from build123d import *

# Parameters (mm, degrees)
SKETCH1_R                                         = 60.625
SKETCH1_R_2                                       = 45
BOSS_EXTRUDE1_DEPTH                               = 4
SKETCH2_R                                         = 49
SKETCH2_R_2                                       = 45
BOSS_EXTRUDE2_DEPTH                               = 52
SKETCH3_W                                         = 8
SKETCH3_H                                         = 38
BOSS_EXTRUDE3_DEPTH                               = 13
SKETCH5_W                                         = 10
SKETCH5_H                                         = 24
CUT_EXTRUDE1_DEPTH                                = 23
SKETCH6_R                                         = 5
CUT_EXTRUDE2_DEPTH                                = 60
SKETCH7_R                                         = 1.3
CUT_EXTRUDE3_DEPTH                                = 7.2
BOSS_EXTRUDE4_DEPTH                               = 4
CSK_FOR_0_FLAT_HEAD_MACHINE_SCREW_100_D           = 1.778
CSK_FOR_0_FLAT_HEAD_MACHINE_SCREW_100_CSINK_D     = 3.0226
CSK_FOR_0_FLAT_HEAD_MACHINE_SCREW_100_CSINK_ANGLE = 100
FILLET1_R                                         = 1


with BuildPart() as part:
    # Sketch1 → Boss-Extrude1 (new body)
    with BuildSketch(Plane(origin=(0, 0, 0), x_dir=(1, 0, 0), z_dir=(0, 1, 0))):
        with Locations(Location((0, 0, 0), (0, 0, 270))):
            Circle(SKETCH1_R)
        with Locations(Location((0, 0, 0), (0, 0, 270))):
            Circle(SKETCH1_R_2, mode=Mode.SUBTRACT)
    extrude(amount=BOSS_EXTRUDE1_DEPTH)

    # Sketch2 → Boss-Extrude2 (add)
    with BuildSketch(Plane(origin=(0, 4, 0), x_dir=(1, 0, 0), z_dir=(0, 1, 0))):
        with Locations(Location((0, 0, 0), (0, 0, 90))):
            Circle(SKETCH2_R)
        with Locations(Location((0, 0, 0), (0, 0, 270))):
            Circle(SKETCH2_R_2, mode=Mode.SUBTRACT)
    extrude(amount=BOSS_EXTRUDE2_DEPTH)

    # Sketch3 → Boss-Extrude3 (add, symmetric)
    with BuildSketch(Plane(origin=(0, 0, 0), x_dir=(0, 0, -1), z_dir=(1, 0, 0))):
        Polygon((-45, 38), (-31.75, 38), (-31.75, 30), (-45, 16.75), align=None)
        with Locations((15.25, 19)):
            Rectangle(SKETCH3_W, SKETCH3_H)
    extrude(amount=BOSS_EXTRUDE3_DEPTH, both=True)


with BuildPart() as boss_extrude3_piece_1:
    # of the separate pieces the step leaves, piece 1, a body of its own (boss_extrude3_pieces)
    add(part.part.solids().sort_by_distance((0, 0, 60.625))[0])

    # Sketch6 → Cut-Extrude2 (cut)
    with BuildSketch(Plane.XY.offset(-11.25)):
        with Locations(Location((0, 14, 0), (0, 0, 90))):
            Circle(SKETCH6_R)
    extrude(amount=-CUT_EXTRUDE2_DEPTH, mode=Mode.SUBTRACT)


with BuildPart() as boss_extrude3_piece_2:
    # of the separate pieces the step leaves, piece 2, a body of its own (boss_extrude3_pieces)
    add(part.part.solids().sort_by_distance((-13, 0, -19.25))[0])

    # Sketch5 → Cut-Extrude1 (cut)
    with BuildSketch(Plane.XY.offset(-11.25)):
        with Locations((0, 17)):
            Rectangle(SKETCH5_W, SKETCH5_H)
    extrude(amount=-CUT_EXTRUDE1_DEPTH, mode=Mode.SUBTRACT)


with BuildPart() as cut_extrude3_tool:
    # Sketch7 → Cut-Extrude3 (new body)
    with BuildSketch(Plane(origin=(0, 38, 0), x_dir=(1, 0, 0), z_dir=(0, 1, 0))):
        with Locations(Location((-5, 13.75, 0), (0, 0, 270))):
            Circle(SKETCH7_R)
        with Locations(Location((5, 13.75, 0), (0, 0, 270))):
            Circle(SKETCH7_R)
        with Locations(Location((5, -34.25, 0), (0, 0, 270))):
            Circle(SKETCH7_R)
        with Locations(Location((-5, -34.25, 0), (0, 0, 270))):
            Circle(SKETCH7_R)
    extrude(amount=-CUT_EXTRUDE3_DEPTH)


with BuildPart() as boss_extrude3_piece_1_1:
    add(boss_extrude3_piece_1.part)

    # Cut-Extrude3: cut by cut_extrude3_tool
    add(cut_extrude3_tool.part, mode=Mode.SUBTRACT)



with BuildPart() as boss_extrude3_piece_2_1:
    add(boss_extrude3_piece_2.part)

    # Cut-Extrude3: cut by cut_extrude3_tool
    add(cut_extrude3_tool.part, mode=Mode.SUBTRACT)


with BuildPart() as boss_extrude3_piece_1_2:
    add(boss_extrude3_piece_1_1.part)

    add(boss_extrude3_piece_2_1.part)  # Boss-Extrude4 merges Boss-Extrude3 piece 2
    # Sketch8 → Boss-Extrude4 (add)
    with BuildSketch(Plane.XZ):
        with BuildLine():
            Line((13, -11.25), (-13, -11.25))
            Line((-13, -11.25), (-37.248431585, -25.249838503))
            ThreePointArc((-37.248431585, -25.249838503), (0, -45), (37.248431585, -25.249838503))
            Line((37.248431585, -25.249838503), (13, -11.25))
        make_face()
        with BuildLine():
            Line((19.516660498, -24.25), (24.906460381, -27.361802413))
            ThreePointArc((24.906460381, -27.361802413), (0, -37), (-24.906460381, -27.361802413))
            Line((-24.906460381, -27.361802413), (-19.516660498, -24.25))
            Line((-19.516660498, -24.25), (19.516660498, -24.25))
        make_face(mode=Mode.SUBTRACT)
    extrude(amount=-BOSS_EXTRUDE4_DEPTH)

    # CSK for #0 Flat Head Machine Screw (100)1 (through all)
    with Locations(Plane(origin=(0, 4, 0), x_dir=(1, 0, 0), z_dir=(0, 1, 0))):
        with Locations((-35, 42), (35, 42), (35, -42), (-35, -42)):
            CounterSinkHole(CSK_FOR_0_FLAT_HEAD_MACHINE_SCREW_100_D / 2, CSK_FOR_0_FLAT_HEAD_MACHINE_SCREW_100_CSINK_D / 2, counter_sink_angle=CSK_FOR_0_FLAT_HEAD_MACHINE_SCREW_100_CSINK_ANGLE)

    # Fillet1
    fillet1_edges = [boss_extrude3_piece_1_2.edges().sort_by_distance(p)[0] for p in [
        (0, 4, 49),
    ]]
    fillet(fillet1_edges, radius=FILLET1_R)


solid = boss_extrude3_piece_1_2.part
Read the model definition and answer for the solid it produces. Units are mm, in the model's axes. A direction names the side the tool comes from. Round coordinates to 2 decimals unless told otherwise and drop trailing zeros. Loops run counter-clockwise (first coordinate to the right, second up) from the corner with the lowest first, then second, coordinate; pieces in that order, holes last.
Q1. Section A-A on y = 20.5 is taken. Write down the section's boundary in (x, z), and give its area (3 significant figures).
Q2. Which of the six approach directions +Z, -Z, +X, -X, +Y, -Y give full straight-line access (tool end or side, diameter ignored) to faces 1 (the face through (0, 9, -47)), 2 (the face through (5, 17, -15)), 3 (the face through (13, 21, -15)), 4 (the face through (-22.2, 2, -25.8))?
Q3. Each of these flat-tipped pins is pushed along its axis until it touches: pin 1 (14.5 mm diameter, centred on x = -6, z = 36.5, fed in from +Y); pin 2 (3.5 mm diameter, centred on y = 24.5, z = 35, fed in from +X); pin 3 (2 mm diameter, centred on y = 17.5, z = 18, fed in from -X). Where does it stop, or does it pass through?
Q4. Determine the mould class of faces 5 (the face through (-36.9, 2, -48.1)), 6 (the face through (22, 56, -40)), 7 (the face through (-13, 21, -15)) for opening direction X: released by +X, released by -X, zero draft, split by the parting line, or undercut.
Q5. Section D-D on y = 47 is taken. Write down the section's boundary in (x, z).
Q6. Section B-B on z = 0 is taken. Write down the section's boundary in (x, y) (3 decimals).
Q7. Section C-C on y = 12.5 is taken. Write down the section's boundary in (x, z).
Q8. Consider probe 1 along Z at (x, y) = (-10.5, 17.5); probe 2 along X at (y, z) = (2.3, -42); probe 3 along Y at (x, z) = (-1, -15.5). Determine where each line is inside the solid, lowest interval first.
Output:
1. outline: circle Ø98 at (0, 0); (-13, -19.25) - (-5, -19.25) - (-5, -11.25) - (-13, -11.25) - close; (5, -19.25) - (13, -19.25) - (13, -11.25) - (5, -11.25) - close; hole (-13, 41.25) - (-13, 43.08) arc R45 ccw (long way) to (13, 43.08) - (13, 41.25) - close
1. area: 1,390 mm2
2. face 1: -Z
2. face 2: none
2. face 3: +Y
2. face 4: +Y, -Y
3. pin 1: stops at y = 38
3. pin 2: stops at x = 35.99
3. pin 3: stops at x = -45.96
4. face 5: split by the parting line
4. face 6: zero draft
4. face 7: undercut
5. outline: circle Ø98 at (0, 0); hole circle Ø90 at (0, 0)
6. outline: (-60.625, 0) - (-45, 0) - (-45, 56) - (-49, 56) - (-49, 5) arc R1 cw to (-50, 4) - (-60.625, 4) - close; (45, 0) - (60.625, 0) - (60.625, 4) - (50, 4) arc R1 cw to (49, 5) - (49, 56) - (45, 56) - close
7. outline: (-13, -19.25) - (-5, -19.25) - (-5, -11.25) - (-13, -11.25) - close; (-4.77, -48.77) - (-4.77, -44.75) arc R45 cw (long way) to (4.77, -44.75) - (4.77, -48.77) arc R49 ccw (long way) to start; (5, -19.25) - (13, -19.25) - (13, -11.25) - (5, -11.25) - close
8. probe 1: z = -47.86 to -43.76, -19.25 to -11.25, 43.76 to 47.86
8. probe 2: x = -43.72 to -35.89, -34.11 to 34.11, 35.89 to 43.72
8. probe 3: y = 0 to 5, 29 to 38
